from build123d import *


with BuildPart() as part:
    # 扫描2: sweep along a path in 草图3
    with BuildLine(Plane(origin=(0, 0, 0), x_dir=(0, 0, -1), z_dir=(1, 0, 0))) as sweep_2_path:
        Line((0, -36.524100396), (-338.88345961, -36.524100396))
        ThreePointArc((-338.88345961, -36.524100396), (-380.294506826, -31.072232602), (-418.88345961, -15.088165001))
        Line((-418.88345961, -15.088165001), (-505.485999988, 34.911834999))
    # 草图2 → 扫描2 (sweep)
    with BuildSketch(Plane.XY):
        Polygon((-41, -55.412292473), (-41, -77.635908318), (41, -77.635908318), (41, -55.412292473), (41, -17.635908318), (41, -5.635908318), (26, -5.635908318), (26, -17.635908318), (16, -17.635908318), (16, -23.635908318), (26, -23.635908318), (26, -67.384306902), (-26, -67.384306902), (-26, -23.635908318), (-16, -23.635908318), (-16, -17.635908318), (-26, -17.635908318), (-26, -5.635908318), (-41, -5.635908318), (-41, -17.635908318), align=None)
    sweep(path=sweep_2_path.line)


solid = part.part
Check sheet for the modelled part. Datum: model origin and axes. Units: mm. A direction names the side the tool comes from. Round coordinates to 2 decimals unless told otherwise and drop trailing zeros. Order: outer loops, then holes, each group sorted by start corner. A loop starts at its lowest first (then second) coordinate and runs counter-clockwise, first axis right, second up.
(1) Cross-section at B-B, the plane z = 44. Enter the section's corners in (x, y), and give its area (3 significant figures).
(2) Draft check along Y on faces 1 (the cylindrical face through (21.07, -18.76, 376.44)), 2 (the flat face through (21.07, 26.62, 453.35)), 3 (the flat face through (-28, -41, 0)). Enter one of: pulls with the +Y half, pulls with the -Y half, needs draft (parallel to the pull), parting line crosses it, or undercut.
(3) Scan lines: probe 1 along Y at (x, z) = (-18.5, 175.5); probe 2 along X at (y, z) = (-19.5, 224.5); probe 3 along X at (y, z) = (-35.5, 72). Record each from-to range of solid material in increasing order.
(4) Go/stop test with flat-tipped pins: P1, Ø24, axis at y = 20.5, z = 367, coming from the +X side; P2, Ø3, axis at x = -19.5, z = 244.5, coming from the +Y side; P3, Ø1, axis at x = -17, y = 40, coming from the -Z side; P4, Ø2, axis at x = -7.5, z = 233.5, coming from the +Y side. Record where each tip stops, or that it passes through.
(5) Cross-section at C-C, the plane x = 33.5. Enter the section's corners in (y, z).
(6) Cross-section at A-A, the plane x = -21. Enter the section's corners in (y, z), and give its area (3 significant figures).
(7) Access from +Z, -Z, +X, -X, +Y, -Y to the whole of each face (thin tool, end or side, straight path). Record for faces 4 (the flat face through (-21, -17.636, 172)), 5 (the cylindrical face through (-0.36, -61.06, 387.61)), 6 (the flat face through (-21.07, 21.423, 456.347)).
Check sheet entries:
1. outline: (-41, -77.64) - (41, -77.64) - (41, -5.64) - (26, -5.64) - (26, -17.64) - (16, -17.64) - (16, -23.64) - (26, -23.64) - (26, -67.38) - (-26, -67.38) - (-26, -23.64) - (-16, -23.64) - (-16, -17.64) - (-26, -17.64) - (-26, -5.64) - (-41, -5.64) - close
1. area: 2,810 mm2
2. face 1: undercut
2. face 2: pulls with the +Y half
2. face 3: needs draft
3. probe 1: y = -77.64 to -67.38, -23.64 to -17.64
3. probe 2: x = -41 to -16, 16 to 41
3. probe 3: x = -41 to -26, 26 to 41
4. P1: passes through
4. P2: stops at y = -17.64
4. P3: stops at z = 475.66
4. P4: stops at y = -67.38
5. outline: (-77.64, 0) - (-5.64, 0) - (-5.64, 338.88) arc R129.11 cw to (11.66, 403.44) - (61.66, 490.04) - (-0.69, 526.04) - (-50.69, 439.44) arc R201.11 ccw to (-77.64, 338.88) - close
6. outline: (-77.64, 0) - (-67.38, 0) - (-67.38, 338.88) arc R190.86 cw to (-41.81, 434.31) - (8.19, 520.92) - (-0.69, 526.04) - (-50.69, 439.44) arc R201.11 ccw to (-77.64, 338.88) - close; (-23.64, 0) - (-17.64, 0) - (-17.64, 338.88) arc R141.11 cw to (1.27, 409.44) - (51.27, 496.04) - (46.07, 499.04) - (-3.93, 412.44) arc R147.11 ccw to (-23.64, 338.88) - close
6. area: 8,640 mm2
7. face 4: -Z, +Y
7. face 5: -Z
7. face 6: none
